```python
from build123d import *

# Parameters (mm, degrees)
ESQUISSE1_W             = 10
ESQUISSE1_H             = 4
BOSS_EXTRU_1_DEPTH      = 2
ESQUISSE2_R             = 0.75
ENL_V_MAT_EXTRU_1_DEPTH = 10
ESQUISSE7_W             = 2.75
ESQUISSE7_H             = 1
ENL_V_MAT_EXTRU_3_DEPTH = 3
ESQUISSE8_W             = 3
ESQUISSE8_H             = 2.75
ENL_V_MAT_EXTRU_5_DEPTH = 1
CONG_1_R                = 1
CONG_2_R                = 0.5
CONG_3_R                = 0.5
CONG_4_R                = 0.3


with BuildPart() as part:
    # Esquisse1 → Boss.-Extru.1 (new body)
    with BuildSketch(Plane(origin=(0, 0, 0), x_dir=(1, 0, 0), z_dir=(0, 1, 0))):
        Rectangle(ESQUISSE1_W, ESQUISSE1_H)
    extrude(amount=BOSS_EXTRU_1_DEPTH)

    # Esquisse2 → Enlèv. mat.-Extru.1 (cut)
    with BuildSketch(Plane(origin=(5, 0, 0), x_dir=(0, 0, -1), z_dir=(1, 0, 0))):
        with Locations((0, 1)):
            Circle(ESQUISSE2_R)
    extrude(amount=-ENL_V_MAT_EXTRU_1_DEPTH, mode=Mode.SUBTRACT)

    # Esquisse7 → Enlèv. mat.-Extru.3 (cut)
    with BuildSketch(Plane.ZY.offset(5)):
        with Locations((-0.625, 1.5)):
            Rectangle(ESQUISSE7_W, ESQUISSE7_H)
    enl_v_mat_extru_3 = extrude(amount=-ENL_V_MAT_EXTRU_3_DEPTH, mode=Mode.SUBTRACT)

    # Symétrie1: Enlèv. mat.-Extru.3 across plane
    add(enl_v_mat_extru_3.mirror(Plane.ZY), mode=Mode.SUBTRACT)

    # Esquisse8 → Enlèv. mat.-Extru.5 (cut)
    with BuildSketch(Plane.XZ):
        with Locations((-1.5, -0.625)):
            Rectangle(ESQUISSE8_W, ESQUISSE8_H)
    enl_v_mat_extru_5 = extrude(amount=-ENL_V_MAT_EXTRU_5_DEPTH, mode=Mode.SUBTRACT)

    # Symétrie3: Enlèv. mat.-Extru.5 across plane
    add(enl_v_mat_extru_5.mirror(Plane.ZY), mode=Mode.SUBTRACT)

    # Congé1
    cong_1_edges = [part.edges().sort_by_distance(p)[0] for p in [
        (-4, 1, -0.75),
        (0, 1, -0.75),
        (4, 1, -0.75),
    ]]
    fillet(cong_1_edges, radius=CONG_1_R)

    # Congé2
    cong_2_edges = [part.edges().sort_by_distance(p)[0] for p in [
        (-4, 1, -2),
        (0, 1, -2),
        (4, 1, -2),
    ]]
    fillet(cong_2_edges, radius=CONG_2_R)

    # Congé3
    cong_3_edges = [part.edges().sort_by_distance(p)[0] for p in [
        (0, 2, -2),
        (0, 2, 2),
    ]]
    fillet(cong_3_edges, radius=CONG_3_R - 0.0001)  # a hair under: the kernel refuses the full size

    # Congé4
    cong_4_edges = [part.edges().sort_by_distance(p)[0] for p in [
        (-2, 1.5, 0.75),
        (2, 1.5, 0.75),
        (-3, 0.5, 0.75),
        (3, 0.5, 0.75),
    ]]
    fillet(cong_4_edges, radius=CONG_4_R)


solid = part.part
```
Work out the finished part from the listing and answer in its coordinate system (mm). A direction names the side the tool comes from. Round coordinates to 2 decimals unless told otherwise and drop trailing zeros. Loops run counter-clockwise (first coordinate to the right, second up) from the corner with the lowest first, then second, coordinate; pieces in that order, holes last. Notation, with made-up numbers: (-19.75, 52.5) -> (-12.75, 52.5) arc R36 ccw to (-12.75, 88.5) -> close; hole circle Ø2 at (57, -36). An arc over 180 degrees is marked (long way). Write each question's results on one line, items separated by ' | '. Start each with the question number.
1. Section D-D (z = 0.1) is taken. Determine the outline of the cut face in (x, y).
2. A tool of negligible diameter and unlimited length cuts with its end or side. For faces 1 (the face through (2, 1.6, -1.1)), 2 (the face through (3, 0.4, -1.1)), 3 (the face through (-3.83, 0.29, 0.24)), 4 (the face through (-2, 1.6, -1.1)), 5 (the face through (0, 2, 0)), from which of +Z, -Z, +X, -X, +Y, -Y can it reach the whole face along a straight path? Write none if from no direction.
3. Section A-A (y = 0.85) is taken. Determine the outline of the cut face in (x, z), plus the area to 3 significant figures.
4. Find the intervals of material crossed by probe 1 along X at (y, z) = (0.4, -1.65); probe 2 along Z at (x, y) = (-1.75, 0.7); probe 3 along Y at (x, z) = (3.5, 0), in increasing order. Write a range as from..to.
5. Section C-C (z = -0.85) is taken. Determine the outline of the cut face in (x, y).
6. For a pull along X with two mould halves and no side action, classify faces 6 (the face through (5, 1, 1)), 7 (the face through (-0.1, 0.8, 0.75)), 8 (the face through (-3, 0.4, -1.1)), 9 (the face through (0.03, 1.72, 0.21)) as +X half, -X half, draft (parallel to the pull), parting line (faces both ways), or undercut.
7. Section B-B (x = 3.5) is taken. Determine the outline of the cut face in (y, z), plus the area to 3 significant figures.
8. Given pin 1 Ø0.5 at (y, z) = (1.5, -0.5) entering from -X, flat-ended and moving along its own axis, determine where the tip first touches the part or whether it passes through.
Evaluation:
1) outline: (-5, 0) -> (-3, 0) -> (-3, 0.26) -> (-5, 0.26) -> close; (-2, 1.74) -> (2, 1.74) -> (2, 2) -> (-2, 2) -> close; (3, 0) -> (5, 0) -> (5, 0.26) -> (3, 0.26) -> close
2) face 1: -Z, +X, +Y, -Y | face 2: -Z, +Y, -Y | face 3: +X, -X, +Y | face 4: -Z, -X, +Y, -Y | face 5: +Z, -Z, +X, -X, +Y
3) outline: (-5, -1.86) -> (-3, -1.86) -> (-3, -0.91) -> (-5, -0.91) -> close; (-5, 0.73) -> (-2.79, 0.73) arc R0.3 cw to (-2.7, 0.75) -> (2.7, 0.75) arc R0.3 cw to (2.79, 0.73) -> (5, 0.73) -> (5, 2) -> (-5, 2) -> close; (3, -1.86) -> (5, -1.86) -> (5, -0.91) -> (3, -0.91) -> close | area: 16.4 mm2
4) probe 1: x = -5..-3, 3..5 | probe 2: z = 0.75..2 | probe 3: y = 0..0.25
5) outline: (-5, 0) -> (-3, 0) -> (-3, 0.81) -> (-5, 0.81) -> close; (-2, 1.19) -> (2, 1.19) -> (2, 2) -> (-2, 2) -> close; (3, 0) -> (5, 0) -> (5, 0.81) -> (3, 0.81) -> close
6) face 6: +X half | face 7: undercut | face 8: undercut | face 9: draft
7) outline: (0, -2) -> (0.5, -2) arc R0.5 ccw to (1, -1.5) -> (1, -1.44) arc R1 ccw to (0.57, -0.62) arc R0.75 cw to (1, 0.75) -> (2, 0.75) -> (2, 1.5) arc R0.5 ccw to (1.5, 2) -> (0, 2) -> close | area: 4.19 mm2
8) pin 1: stops at x = -2
